Input: part model. Units: mm. Frame: model coordinates. Give positions to 0.01 mm unless a question says otherwise; leave off trailing zeros. Order: outer loops, then holes, each group sorted by start corner. A loop starts at its lowest first (then second) coordinate and runs counter-clockwise, first axis right, second up. Notation, with made-up numbers: (-28.5, -33) - (9.5, -33) arc R16 cw to (9.5, -5) - close; hole circle Ø2 at (-5, 45.25). An arc over 180 degrees is marked (long way). Use a Markdown table: item, result.
from build123d import *

# Parameters (mm, degrees)
SWEEP1_PROFILE_R    = 6.35
SKETCH20_R          = 3.175
BOSS_EXTRUDE3_DEPTH = 38.1


with BuildPart() as part:
    # Sweep1: sweep along a path in Sketch1
    with BuildLine(Plane.XY) as sweep1_path:
        Line((0, 0), (527.05, 0))
        Line((527.05, 0), (527.05, 50.8))
        Line((527.05, 50.8), (831.85, 50.8))
    # Sweep1 profile (on start of the path) → Sweep1 (sweep)
    with BuildSketch(Plane.YZ):
        Circle(SWEEP1_PROFILE_R)
    sweep(path=sweep1_path.line, transition=Transition.RIGHT)

    # Sketch20 → Boss-Extrude3 (add)
    with BuildSketch(Plane(origin=(831.85, 0, 0), x_dir=(0, 0, -1), z_dir=(1, 0, 0))):
        with Locations(Location((0, 50.8, 0), (0, 0, 270))):
            Circle(SKETCH20_R)
    extrude(amount=BOSS_EXTRUDE3_DEPTH)


solid = part.part
1. Material intervals for line 1 along X through (y, z) = (24, 0.75); line 2 along Y through (x, z) = (193, -5.5); line 3 along Y through (x, z) = (608, 0.75), sorted ascending.
Response:
| item | result |
|---|---|
| line 1 | x = 520.74 to 533.36 |
| line 2 | y = -3.17 to 3.17 |
| line 3 | y = 44.49 to 57.11 |
2. Section query A-A (z = 0). Return loops of the section in (x, y) (3 decimals).
Response:
| item | result |
|---|---|
| outline | (0, -6.35) - (533.4, -6.35) - (533.4, 44.45) - (831.85, 44.45) - (831.85, 47.625) - (869.95, 47.625) - (869.95, 53.975) - (831.85, 53.975) - (831.85, 57.15) - (520.7, 57.15) - (520.7, 6.35) - (0, 6.35) - close |
3. Pin query (flat end, axial travel): pin 1 (6 mm diameter, centred on y = 38, z = 0, fed in from +X); pin 2 (5 mm diameter, centred on x = 181, z = 4.5, fed in from -Y); pin 3 (6 mm diameter, centred on y = 48.5, z = -4.5, fed in from -X); pin 4 (6.5 mm diameter, centred on y = 48, z = -2.5, fed in from +X). Return the tip coordinate at first contact, or that it passes through.
Response:
| item | result |
|---|---|
| pin 1 | stops at x = 533.4 |
| pin 2 | stops at y = -6.03 |
| pin 3 | stops at x = 520.88 |
| pin 4 | stops at x = 869.95 |
4. Section query B-B (y = 35). Return loops of the section in (x, z).
Response:
| item | result |
|---|---|
| outline | circle Ø12.7 at (527.05, 0) |
5. Section query C-C (x = 248). Return loops of the section in (y, z), then the cut area to 3 significant figures.
Response:
| item | result |
|---|---|
| outline | circle Ø12.7 at (0, 0) |
| area | 127 mm^2 |
